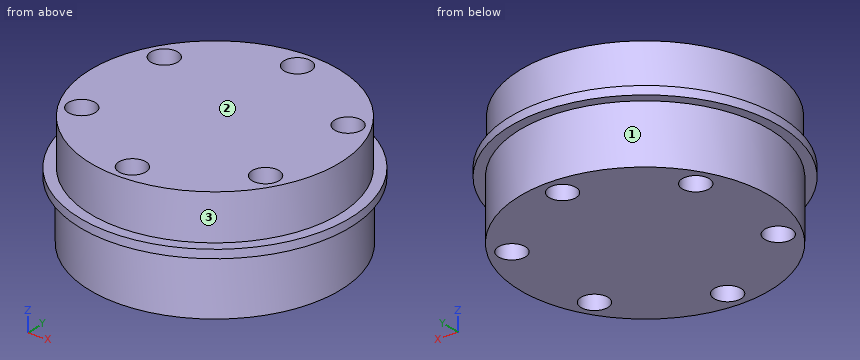
from build123d import *

# Parameters (mm, degrees)
SKETCH_1_R          = 14.75
EXTRUDE_1_DEPTH     = 5.4
SKETCH_3_R          = 16
EXTRUDE_2_DEPTH     = 1
SKETCH_4_R          = 14.85
EXTRUDE_3_DEPTH     = 7
SKETCH_2_R          = 1.6
CUT_EXTRUDE_2_DEPTH = 27.297528401


with BuildPart() as part:
    # 草图1 → 凸台-拉伸1 (new body)
    with BuildSketch(Plane.XY):
        with Locations(Location((0, 0, 0), (0, 0, 180))):
            Circle(SKETCH_1_R)
    extrude(amount=EXTRUDE_1_DEPTH)

    # 草图3 → 凸台-拉伸2 (add)
    with BuildSketch(Plane(origin=(0, 0, 0), x_dir=(-1, 0, 0), z_dir=(0, 0, -1))):
        Circle(SKETCH_3_R)
    extrude(amount=EXTRUDE_2_DEPTH)

    # 草图4 → 凸台-拉伸3 (add)
    with BuildSketch(Plane(origin=(0, 0, -1), x_dir=(-1, 0, 0), z_dir=(0, 0, -1))):
        Circle(SKETCH_4_R)
    extrude(amount=EXTRUDE_3_DEPTH)

    # 草图2 → 切除-拉伸2 (cut, through all)
    with BuildSketch(Plane(origin=(0, 0, 5.4), x_dir=(-1, 0, 0), z_dir=(0, 0, -1))):
        with Locations((10.825317547, -6.25)):
            Circle(SKETCH_2_R)
        with Locations((-10.825317547, 6.25)):
            Circle(SKETCH_2_R)
        with Locations((-10.825317547, -6.25)):
            Circle(SKETCH_2_R)
        with Locations((0, -12.5)):
            Circle(SKETCH_2_R)
        with Locations((10.825317547, 6.25)):
            Circle(SKETCH_2_R)
        with Locations((0, 12.5)):
            Circle(SKETCH_2_R)
    extrude(amount=CUT_EXTRUDE_2_DEPTH, mode=Mode.SUBTRACT)


solid = part.part
The model under review builds one solid part; all positions refer to its coordinate system, in mm. Face numbers are marked on the shaded views. A direction names the side the tool comes from. Give positions to 0.01 mm unless a question says otherwise; leave off trailing zeros. Write each loop counter-clockwise with the first axis right and the second up, starting at its lowest first coordinate (ties: lowest second). Pieces come first, ordered by that corner, then holes. Notation, with made-up numbers: M 15,66 L 41,66 A32 cw 41,103 Z; hole C 24,34.5 d5. An arc over 180 degrees is marked long. One line per question, with ' | ' between items. Start each with the question number.
Item 1: For pin 1 (5 mm diameter, centred on x = 0, z = -6, fed in from -Y); pin 2 (5 mm diameter, centred on x = -12.5, z = -1.5, fed in from -Y); pin 3 (8 mm diameter, centred on y = 11, z = -5, fed in from -X), all flat-tipped, find the tip position at first contact; note any pin that passes through.
Item 2: We need section C-C on y = -13.5. Write out the cut boundary in (x, z), plus the area to 3 significant figures.
Item 3: Wall thickness on line 1 (Y direction, x = 0, z = -1.5); line 2 (X direction, y = 6, z = -5.25); line 3 (X direction, y = 6.25, z = -1.75): over which ranges is each line inside the solid? List them lowest first. Write a range as from..to.
Item 4: For the marked faces 1, 2 and 3, list the 3-axis set-ups (+Z, -Z, +X, -X, +Y, -Y) from which the entire face can be reached by the end or side of a thin tool; tool diameter is ignored.
Item 5: We need section D-D on x = -1. Write out the cut boundary in (y, z).
Item 6: We need section A-A on z = 2.75. Write out the cut boundary in (x, y), plus the area to 3 significant figures.
Item 7: We need section B-B on y = -6.25. Write out the cut boundary in (x, z).
Results found:
1) pin 1: stops at y = -14.85 | pin 2: stops at y = -12.45 | pin 3: stops at x = -13.1
2) outline: M -8.59,-1 L -6.19,-1 L -6.19,-8 L -1.25,-8 L -1.25,5.4 L -5.94,5.4 L -5.94,0 L -8.59,0 Z; M 1.25,-8 L 6.19,-8 L 6.19,-1 L 8.59,-1 L 8.59,0 L 5.94,0 L 5.94,5.4 L 1.25,5.4 Z | area: 134 mm2
3) line 1: y = -14.85..-14.1, -10.9..10.9, 14.1..14.85 | line 2: x = -13.58..-12.41, -9.24..9.24, 12.41..13.58 | line 3: x = -13.47..-12.43, -9.23..9.23, 12.43..13.47
4) face 1: -Z | face 2: +Z, +X, -X, +Y, -Y | face 3: +Z
5) outline: M -15.97,-1 L -14.82,-1 L -14.82,-8 L -13.75,-8 L -13.75,5.4 L -14.72,5.4 L -14.72,0 L -15.97,0 Z; M -11.25,-8 L 11.25,-8 L 11.25,5.4 L -11.25,5.4 Z; M 13.75,-8 L 14.82,-8 L 14.82,-1 L 15.97,-1 L 15.97,0 L 14.72,0 L 14.72,5.4 L 13.75,5.4 Z
6) outline: C 0,0 d29.5; hole C -10.83,-6.25 d3.2; hole C -10.83,6.25 d3.2; hole C 0,-12.5 d3.2; hole C 0,12.5 d3.2; hole C 10.83,-6.25 d3.2; hole C 10.83,6.25 d3.2 | area: 635 mm2
7) outline: M -14.73,-1 L -13.47,-1 L -13.47,-8 L -12.43,-8 L -12.43,5.4 L -13.36,5.4 L -13.36,0 L -14.73,0 Z; M -9.23,-8 L 9.23,-8 L 9.23,5.4 L -9.23,5.4 Z; M 12.43,-8 L 13.47,-8 L 13.47,-1 L 14.73,-1 L 14.73,0 L 13.36,0 L 13.36,5.4 L 12.43,5.4 Z
